Source: CAD feature listing. Evaluate the final solid. Frame: model axes, mm. A direction names the side the tool comes from. Give positions to 0.01 mm unless a question says otherwise; leave off trailing zeros. Loops run counter-clockwise (first coordinate to the right, second up) from the corner with the lowest first, then second, coordinate; pieces in that order, holes last. Notation, with made-up numbers: (-10.5, 63.25) -> (2.5, 63.25) arc R7 ccw to (2.5, 70.25) -> close; hole circle Ø9 at (51, 4.5). An arc over 180 degrees is marked (long way). Return JSON: item names as keys, results as strings. Group by question number.
(1) Pin query (flat end, axial travel): pin 1 (0.5 mm diameter, centred on x = 16, z = -0.5, fed in from -Y); pin 2 (2 mm diameter, centred on x = -2, z = 6, fed in from -Y); pin 3 (0.5 mm diameter, centred on x = -14, z = 0, fed in from +Y). Return the tip coordinate at first contact, or that it passes through.
(2) Ray query, line 1 (Z direction, x = 15.5, y = -1.55); line 2 (Z direction, x = -14.25, y = 10.5); line 3 (Y direction, x = 11, z = -3.25). Return the intervals inside material, ascending. Write a range as from..to.
(3) Cut plane B-B on y = 12.5. Return loops of the section in (x, z).
(4) Access query for faces 4 (the face through (-15.226, 12.27, -0.217)), 5 (the face through (16.382, -0.625, -0.472)), 6 (the face through (-14.75, 6, 2)), 7 (the face through (-11.75, 14, 2)), 8 (the face through (13, 8, -4)). Directions: +Z, -Z, +X, -X, +Y, -Y. A direction counts if a zero-diameter tool reaches every point of the face in a straight line with its end or side. Return the directions, or none.
(5) Draft query along X for faces 1 (the face through (17.91, 9.63, 0.11)), 2 (the face through (-14.75, 6, -4)), 3 (the face through (15.5, -3, 1.4)). Return one class per face: released by +X, released by -X, zero draft, split by the parting line, or undercut.
(6) Cut plane D-D on y = 6.5. Return loops of the section in (x, z).
(7) Cut plane A-A on x = 0. Return loops of the section in (y, z).
(8) Cut plane C-C on z = -5.5. Return loops of the section in (x, y) (3 decimals), then the cut area to 3 significant figures.
```python
from build123d import *

# Parameters (mm, degrees)
ESBO_O1_W                = 40
ESBO_O1_H                = 16
RESSALTO_EXTRUS_O1_DEPTH = 2
ESBO_O1_4_W              = 8.25
ESBO_O1_4_H              = 16
ESBO_O1_4_R              = 1
RESSALTO_EXTRUS_O2_DEPTH = 19
ESBO_O2_R                = 3.3
ESBO_O2_R_2              = 1
RESSALTO_EXTRUS_O3_DEPTH = 3
CORTE_EXTRUS_O1_DEPTH    = 32.890437438
CORTE_EXTRUS_O3_DEPTH    = 12
CORTE_EXTRUS_O4_DEPTH    = 12
CHANFRO1_SIZE            = 3
CORTE_EXTRUS_O5_START    = -6
ESBO_O7_R                = 1
CORTE_EXTRUS_O5_DEPTH    = 6


with BuildPart() as part:
    # Esboço1 → Ressalto-extrusão1 (new body)
    with BuildSketch(Plane(origin=(0, 0, 0), x_dir=(1, 0, 0), z_dir=(0, 1, 0))):
        Rectangle(ESBO_O1_W, ESBO_O1_H)
    extrude(amount=RESSALTO_EXTRUS_O1_DEPTH)

    # Esboço1<4> → Ressalto-extrusão2 (add)
    # profile 1 of 2: a face of its own
    with BuildSketch(Plane(origin=(0, 0, 0), x_dir=(1, 0, 0), z_dir=(0, 1, 0))):
        with Locations((-15.875, 0)):
            Rectangle(ESBO_O1_4_W, ESBO_O1_4_H)
        with Locations(Location((-14.25, 0, 0), (0, 0, 270))):
            Circle(ESBO_O1_4_R, mode=Mode.SUBTRACT)
    # profile 2 of 2: a face of its own
    with BuildSketch(Plane(origin=(0, 0, 0), x_dir=(1, 0, 0), z_dir=(0, 1, 0))):
        with Locations((15.875, 0)):
            Rectangle(ESBO_O1_4_W, ESBO_O1_4_H)
        with Locations(Location((14.25, 0, 0), (0, 0, 270))):
            Circle(ESBO_O1_4_R, mode=Mode.SUBTRACT)
    extrude(amount=RESSALTO_EXTRUS_O2_DEPTH)

    # Esboço2 → Ressalto-extrusão3 (add)
    # profile 1 of 3: a face of its own
    with BuildSketch(Plane.XZ):
        with Locations(Location((0, 0, 0), (0, 0, 90))):
            Circle(ESBO_O2_R)
        with Locations(Location((0, 0, 0), (0, 0, 270))):
            Circle(ESBO_O2_R_2, mode=Mode.SUBTRACT)
    # profile 2 of 3: a face of its own
    with BuildSketch(Plane.XZ):
        with Locations(Location((-15.5, 0, 0), (0, 0, 90))):
            Circle(ESBO_O2_R)
        with Locations(Location((-15.5, 0, 0), (0, 0, 270))):
            Circle(ESBO_O2_R_2, mode=Mode.SUBTRACT)
    # profile 3 of 3: a face of its own
    with BuildSketch(Plane.XZ):
        with Locations(Location((15.5, 0, 0), (0, 0, 90))):
            Circle(ESBO_O2_R)
        with Locations(Location((15.5, 0, 0), (0, 0, 270))):
            Circle(ESBO_O2_R_2, mode=Mode.SUBTRACT)
    extrude(amount=RESSALTO_EXTRUS_O3_DEPTH)

    # Esboço3 → Corte-extrusão1 (cut, through all)
    with BuildSketch(Plane.XY.offset(8)):
        Polygon((15.875, 19), (20, 0), (20, 19), align=None)
        Polygon((-20, 0), (-15.875, 19), (-20, 19), align=None)
    extrude(amount=-CORTE_EXTRUS_O1_DEPTH, mode=Mode.SUBTRACT)

    # Esboço4 → Corte-extrusão3 (cut)
    with BuildSketch(Plane(origin=(0, 0, -8), x_dir=(-1, 0, 0), z_dir=(0, 0, -1))):
        Polygon((14.75, 8), (11.75, 13), (11.75, 5), (14.75, 5), align=None)
    extrude(amount=-CORTE_EXTRUS_O3_DEPTH, mode=Mode.SUBTRACT)

    # Esboço6 → Corte-extrusão4 (cut)
    with BuildSketch(Plane.XY.offset(8)):
        Polygon((14.75, 8), (11.75, 13), (11.75, 5), (14.75, 5), align=None)
    extrude(amount=-CORTE_EXTRUS_O4_DEPTH, mode=Mode.SUBTRACT)

    # Chanfro1
    # the kernel refuses this chamfer: 3 mm, written as the material it takes off along each edge
    with BuildSketch(Plane(origin=(11.75, 5, 15.715048964), x_dir=(-0.027495876610586202, -0.9996219169112968, 0), z_dir=(0, 0, -1))) as chanfro1_piece_1_section:
        Polygon((CHANFRO1_SIZE * 0.999621916911, -CHANFRO1_SIZE * 0.0274958766106), (-CHANFRO1_SIZE * 0.0274958766106, -CHANFRO1_SIZE * 0.999621916911), (0, 0), align=None)
    chanfro1_piece_1 = extrude(amount=19.715048964, mode=Mode.PRIVATE)
    chanfro1_piece_1 = split(chanfro1_piece_1, bisect_by=Plane(origin=(12.737731783, 2, 5.857524482), z_dir=(0, 1, 0)), keep=Keep.TOP, mode=Mode.PRIVATE)
    chanfro1_piece_1 = split(chanfro1_piece_1, bisect_by=Plane(origin=(14.75, 4.012268217, 5.857524482), z_dir=(-1, 0, 0)), keep=Keep.TOP, mode=Mode.PRIVATE)
    add(chanfro1_piece_1, mode=Mode.SUBTRACT)
    with BuildSketch(Plane(origin=(-11.75, 5, -15.715048964), x_dir=(0.027495876610586202, -0.9996219169112968, 0), z_dir=(0, 0, 1))) as chanfro1_piece_2_section:
        Polygon((CHANFRO1_SIZE * 0.999621916911, -CHANFRO1_SIZE * 0.0274958766106), (-CHANFRO1_SIZE * 0.0274958766106, -CHANFRO1_SIZE * 0.999621916911), (0, 0), align=None)
    chanfro1_piece_2 = extrude(amount=19.715048964, mode=Mode.PRIVATE)
    chanfro1_piece_2 = split(chanfro1_piece_2, bisect_by=Plane(origin=(-12.737731783, 2, -5.857524482), z_dir=(0, 1, 0)), keep=Keep.TOP, mode=Mode.PRIVATE)
    chanfro1_piece_2 = split(chanfro1_piece_2, bisect_by=Plane(origin=(-14.75, 4.012268217, -5.857524482), z_dir=(1, 0, 0)), keep=Keep.TOP, mode=Mode.PRIVATE)
    add(chanfro1_piece_2, mode=Mode.SUBTRACT)

    # Esboço7 → Corte-extrusão5 (cut)
    with BuildSketch(Plane.XZ.offset(3).offset(CORTE_EXTRUS_O5_START)):
        with Locations(Location((0, 0, 0), (0, 0, 90))):
            Circle(ESBO_O7_R)
        with Locations(Location((-15.5, 0, 0), (0, 0, 51.317812547))):
            Circle(ESBO_O7_R)
        with BuildLine():
            ThreePointArc((14.5, 0), (15.5, -1), (16.5, 0))
            Line((16.5, 0), (14.5, 0))
        make_face()
        with BuildLine():
            Line((14.5, 0), (16.5, 0))
            ThreePointArc((16.5, 0), (15.5, 1), (14.5, 0))
        make_face()
    extrude(amount=CORTE_EXTRUS_O5_DEPTH, mode=Mode.SUBTRACT)


solid = part.part
```
Answers:
{
 "1": {"pin 1": "y = 3", "pin 2": "y = 0", "pin 3": "y = 2"},
 "2": {"line 1": "-3.3..-1, 1..3.3", "line 2": "-8..-1, 1..8", "line 3": "0..2"},
 "3": {"outline": "(-17.29, -8) -> (-12.05, -8) -> (-12.05, 4) -> (-11.75, 4) -> (-11.75, 8) -> (-17.29, 8) -> close; (11.75, -8) -> (17.29, -8) -> (17.29, 8) -> (12.05, 8) -> (12.05, -4) -> (11.75, -4) -> close; hole circle Ø2 at (-14.25, 0); hole circle Ø2 at (14.25, 0)"},
 "4": {"face 4": "+Y", "face 5": "-Y", "face 6": "-Z", "face 7": "+Z, -Z, +Y", "face 8": "+Z"},
 "5": {"face 1": "released by +X", "face 2": "undercut", "face 3": "zero draft"},
 "6": {"outline": "(-18.59, -8) -> (-14.75, -8) -> (-14.75, -0.87) arc R1 cw to (-14.75, 0.87) -> (-14.75, 4) -> (-11.75, 4) -> (-11.75, 8) -> (-18.59, 8) -> close; (11.75, -8) -> (18.59, -8) -> (18.59, 8) -> (14.75, 8) -> (14.75, 0.87) arc R1 cw to (14.75, -0.87) -> (14.75, -4) -> (11.75, -4) -> close"},
 "7": {"outline": "(-3, -3.3) -> (0, -3.3) -> (0, -8) -> (2, -8) -> (2, -1) -> (-3, -1) -> close; (-3, 1) -> (2, 1) -> (2, 8) -> (0, 8) -> (0, 3.3) -> (-3, 3.3) -> close"},
 "8": {"outline": "(-20, 0) -> (20, 0) -> (15.875, 19) -> (11.75, 19) -> (11.75, 2) -> (-11.75, 2) -> (-14.75, 5) -> (-14.75, 8) -> (-11.75, 13) -> (-11.75, 19) -> (-15.875, 19) -> close", "area": "261 mm²"}
}
